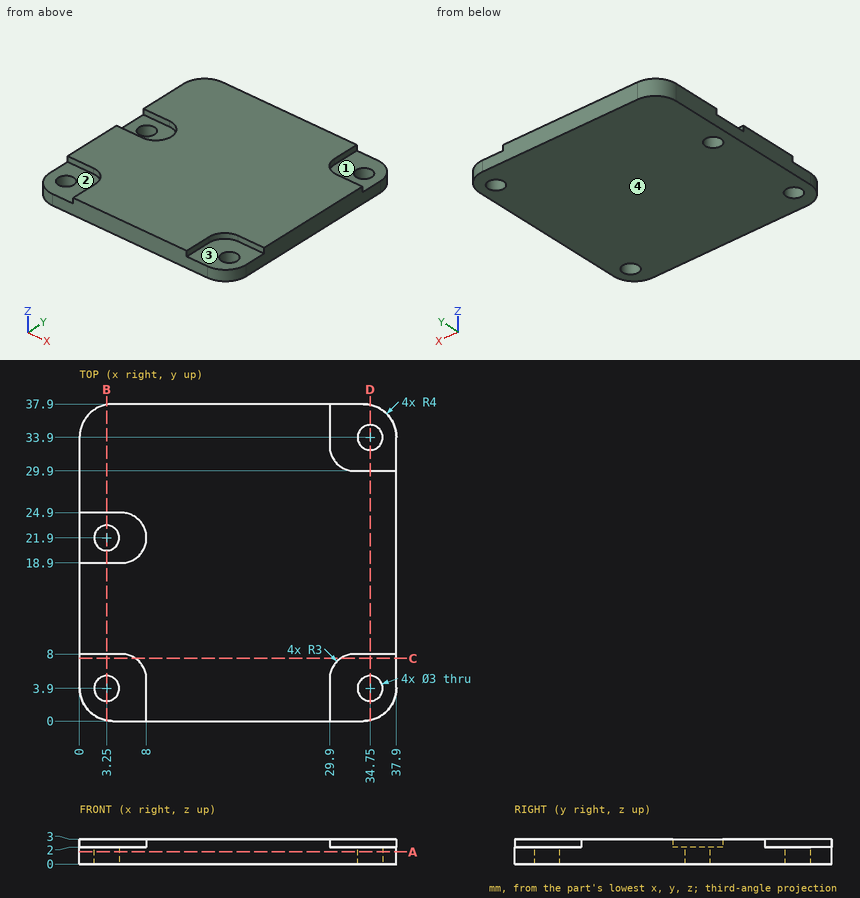
Could you check a few things on this drawing? It's one solid part, dimensions in mm from its lowest x, y, z. A direction names the side the tool comes from. Round coordinates to 2 decimals unless told otherwise and drop trailing zeros. Loops run counter-clockwise (first coordinate to the right, second up) from the corner with the lowest first, then second, coordinate; pieces in that order, holes last.
Q1. Please list where these lines run through material, in increasing order: L1, parallel to Y at x = 34.75, z = 1.35; L2, parallel to Y at x = 3.25, z = 0.7; L3, parallel to X at y = 33, z = 1.2.
Q2. I want a section at A-A (z = 1.45). Write out the boundary of the cut face in (x, y), and give its area (3 significant figures).
Q3. I want a section at C-C (y = 7.5). Write out the boundary of the cut face in (x, z), and give its area (3 significant figures).
Q4. For P1, Ø0.8, axis at x = 3.5, z = 2.5, coming from the -Y side; P2, Ø1.1, axis at y = 3.5, z = 2.5, coming from the +X side; P3, Ø2.5, axis at x = 34.75, y = 3.9, coming from the +Z side; P4, Ø6.5, axis at x = 34.5, y = 33.5, coming from the +Z side, each with a flat end and sliding along its axis, tell me the tip position at first contact or that it passes through.
Q5. I want a section at B-B (x = 3.25). Write out the boundary of the cut face in (y, z), and give its area (3 significant figures).
Q6. On a 3-axis mill with a long thin cutter (end or side, diameter ignored), from which of +Z, -Z, +X, -X, +Y, -Y can I reach the whole of each face in a straight line? I mean the marked faces 1, 2, 3 and 4. Say none if no direction works.
Q7. I want a section at D-D (x = 34.75). Write out the boundary of the cut face in (y, z).
Answer below:
1. L1: y = 0.09 to 2.4, 5.4 to 32.4, 35.4 to 37.81
1. L2: y = 0.07 to 2.4, 5.4 to 20.4, 23.4 to 37.83
1. L3: x = 0 to 33.55, 35.95 to 37.9
2. outline: (0, 4) arc R4 ccw to (4, 0) - (33.9, 0) arc R4 ccw to (37.9, 4) - (37.9, 33.9) arc R4 ccw to (33.9, 37.9) - (4, 37.9) arc R4 ccw to (0, 33.9) - close; hole circle Ø3 at (3.25, 3.9); hole circle Ø3 at (3.25, 21.9); hole circle Ø3 at (34.75, 3.9); hole circle Ø3 at (34.75, 33.9)
2. area: 1,390 mm2
3. outline: (0, 0) - (37.9, 0) - (37.9, 2) - (31.24, 2) - (31.24, 3) - (6.66, 3) - (6.66, 2) - (0, 2) - close
3. area: 100 mm2
4. P1: stops at y = 8
4. P2: stops at x = 37.89
4. P3: passes through
4. P4: stops at z = 2
5. outline: (0.07, 0) - (2.4, 0) - (2.4, 2) - (0.07, 2) - close; (5.4, 0) - (20.4, 0) - (20.4, 2) - (18.9, 2) - (18.9, 3) - (8, 3) - (8, 2) - (5.4, 2) - close; (23.4, 0) - (37.83, 0) - (37.83, 3) - (24.9, 3) - (24.9, 2) - (23.4, 2) - close
5. area: 87.3 mm2
6. face 1: +Z, +X, +Y
6. face 2: +Z, -X, -Y
6. face 3: +Z, +X, -Y
6. face 4: -Z, +X, -X, +Y, -Y
7. outline: (0.09, 0) - (2.4, 0) - (2.4, 2) - (0.09, 2) - close; (5.4, 0) - (32.4, 0) - (32.4, 2) - (29.9, 2) - (29.9, 3) - (8, 3) - (8, 2) - (5.4, 2) - close; (35.4, 0) - (37.81, 0) - (37.81, 2) - (35.4, 2) - close
